Read the model definition and answer for the solid it produces. Units are mm, in the model's axes. A direction names the side the tool comes from. Give positions to 0.01 mm unless a question says otherwise; leave off trailing zeros. Loops run counter-clockwise (first coordinate to the right, second up) from the corner with the lowest first, then second, coordinate; pieces in that order, holes last. Notation, with made-up numbers: (88, -25.5) -> (129, -25.5) arc R23 cw to (129, -3.5) -> close; hole circle Ø2 at (-40, -36.5). An arc over 180 degrees is marked (long way). Answer as CSV lines item,"result". Start each with the question number.
```python
from build123d import *

# Parameters (mm, degrees)
SKETCH1_W                       = 28.575
SKETCH1_H                       = 50.8
BOSS_EXTRUDE1_DEPTH             = 6.35
F_10_32_TAPPED_HOLE1_AT_2_COUNT = 2
F_10_32_TAPPED_HOLE1_AT_2_PITCH = 19.05
F_1_4_0_25_DIAMETER_HOLE1_D     = 6.35
F_1_4_0_25_DIAMETER_HOLE1_DEPTH = 10.668
F_1_4_0_25_DIAMETER_HOLE1_TIP   = 1.907732465
CHAMFER1_SIZE                   = 1.905
CUT_EXTRUDE1_DEPTH              = 7.35
FILLET1_R                       = 6.35


with BuildPart() as part:
    # Sketch1 → Boss-Extrude1 (new body)
    with BuildSketch(Plane.XY):
        Rectangle(SKETCH1_W, SKETCH1_H)
    extrude(amount=BOSS_EXTRUDE1_DEPTH)

    # Sketch3 → #10-32 Tapped Hole1 (revolve, cut)
    with BuildSketch(Plane(origin=(-9.525, 25.4, 3.175), x_dir=(0, 0, 1), z_dir=(1, 0, 0))):
        Polygon((0, 0), (0, 10.865317848), (2.0193, 9.652), (2.0193, 0), align=None)
    f_10_32_tapped_hole1 = revolve(axis=Axis((-9.525, 31.75, 3.175), (0, -1, 0)), mode=Mode.SUBTRACT)

    # #10-32 Tapped Hole1 at 2: #10-32 Tapped Hole1 ×2
    with Locations(*[(i * F_10_32_TAPPED_HOLE1_AT_2_PITCH, 0, 0) for i in range(1, F_10_32_TAPPED_HOLE1_AT_2_COUNT)]):
        add(f_10_32_tapped_hole1, mode=Mode.SUBTRACT)

    # Mirror1: #10-32 Tapped Hole1 across plane
    add(f_10_32_tapped_hole1.mirror(Plane.ZX), mode=Mode.SUBTRACT)

    # Mirror1 copy 1 sketch → Mirror1 copy 1 (revolve, cut)
    with BuildSketch(Plane(origin=(9.525, -25.4, 3.175), x_dir=(0, 0, 1), z_dir=(1, 0, 0))):
        Polygon((0, 0), (0, -10.865317848), (2.0193, -9.652), (2.0193, 0), align=None)
    revolve(axis=Axis((9.525, -31.75, 3.175), (0, -1, 0)), mode=Mode.SUBTRACT)

    # 1/4 (0.25) Diameter Hole1
    with Locations(Plane.XY.offset(6.35)):
        with Locations((0, 0)):
            Hole(F_1_4_0_25_DIAMETER_HOLE1_D / 2, depth=F_1_4_0_25_DIAMETER_HOLE1_DEPTH)
            with Locations((0, 0, -(F_1_4_0_25_DIAMETER_HOLE1_DEPTH + F_1_4_0_25_DIAMETER_HOLE1_TIP / 2))):  # 118° drill point
                Cone(0, F_1_4_0_25_DIAMETER_HOLE1_D / 2, F_1_4_0_25_DIAMETER_HOLE1_TIP, mode=Mode.SUBTRACT)

    # Chamfer1
    chamfer1_edges = [part.edges().sort_by_distance(p)[0] for p in [
        (3.175, 0, 0),
        (3.175, 0, 6.35),
    ]]
    chamfer(chamfer1_edges, length=CHAMFER1_SIZE)

    # Sketch6 → Cut-Extrude1 (cut, through all)
    with BuildSketch(Plane.XY.offset(6.35)):
        with BuildLine():
            Line((-14.2875, 19.05), (-14.2875, -19.05))
            ThreePointArc((-14.2875, -19.05), (-7.9375, 0), (-14.2875, 19.05))
        make_face()
        with BuildLine():
            Line((14.2875, -19.05), (14.2875, 19.05))
            ThreePointArc((14.2875, 19.05), (7.9375, 0), (14.2875, -19.05))
        make_face()
        with BuildLine():
            Line((-4.7625, 25.4), (4.7625, 25.4))
            ThreePointArc((4.7625, 25.4), (0, 20.6375), (-4.7625, 25.4))
        make_face()
        with BuildLine():
            Line((-4.7625, -25.4), (4.7625, -25.4))
            ThreePointArc((4.7625, -25.4), (0, -20.6375), (-4.7625, -25.4))
        make_face()
    extrude(amount=-CUT_EXTRUDE1_DEPTH, mode=Mode.SUBTRACT)

    # Fillet1
    fillet1_edges = [part.edges().sort_by_distance(p)[0] for p in [
        (-14.2875, 19.05, 3.175),
        (-14.2875, -19.05, 3.175),
        (14.2875, -19.05, 3.175),
        (14.2875, 19.05, 3.175),
    ]]
    fillet(fillet1_edges, radius=FILLET1_R)


solid = part.part
```
(1) Find the intervals of material crossed by line 1 along Y through (x, z) = (0, 2) (1 decimal); line 2 along X through (y, z) = (-1, 1.75); line 3 along Y through (x, z) = (-12, 5.75), in increasing order. Write a range as from..to.
(2) Find section C-C on y = 19. Write down the section's boundary in (x, z) (3 decimals).
(3) Find section D-D on y = -13. Write down the section's boundary in (x, z), then the cut area to 3 significant figures.
(4) A tool of negligible diameter and unlimited length cuts with its end or side. For faces 4 (the face through (-7.554, -20.642, 2.737)), 5 (the face through (14.01, -19.2, 3.13)), 6 (the face through (-14.288, -23, 3)), 7 (the face through (-14.01, 19.2, 3.13)), 8 (the face through (11.496, 20.642, 2.737)), from which of +Z, -Z, +X, -X, +Y, -Y can it reach the whole face along a straight path? Write none if from no direction.
(5) The mould has two halves that part along X. Classify faces 1 (the face through (11.496, -20.642, 2.737)), 2 (the face through (9, 25.4, 1)), 3 (the face through (-14.025, -19.252, 3.131)): pulls with the +X half, pulls with the -X half, needs draft (parallel to the pull), parting line crosses it, or undercut.
(6) Each of these flat-tipped pins is pushed along its axis until it touches: P1, Ø3, axis at x = 9.525, z = 3.175, coming from the -Y side; P2, Ø3.5, axis at x = 9.525, z = 3.175, coming from the -Y side; P3, Ø2.5, axis at x = -9.525, z = 3.175, coming from the +Y side. Where does it stop, or does it pass through?
Answer block:
1,line 1,"y = -20.6..-3.2, 3.2..20.6"
1,line 2,"x = -7.95..-3.18, 3.18..7.95"
1,line 3,"y = -25.4..-15.54, 15.54..25.4"
2,outline,"(-13.944, 0) -> (13.944, 0) -> (13.944, 6.35) -> (-13.944, 6.35) -> close; hole circle Ø4.039 at (-9.525, 3.175); hole circle Ø4.039 at (9.525, 3.175)"
3,outline,"(-10.72, 0) -> (10.72, 0) -> (10.72, 6.35) -> (-10.72, 6.35) -> close"
3,area,"136 mm2"
4,face 4,"-Y"
4,face 5,"+Z, -Z, +X"
4,face 6,"+Z, -Z, -X, +Y, -Y"
4,face 7,"+Z, -Z, -X"
4,face 8,"+Y"
5,face 1,"undercut"
5,face 2,"needs draft"
5,face 3,"pulls with the -X half"
6,P1,"stops at y = -15.44"
6,P2,"stops at y = -15.59"
6,P3,"stops at y = 15.29"
